Verification items for the finished model (mm, model axes). A direction names the side the tool comes from. Coordinates: 2 decimals unless noted, no trailing zeros. Write each loop counter-clockwise with the first axis right and the second up, starting at its lowest first coordinate (ties: lowest second). Pieces come first, ordered by that corner, then holes. Notation, with made-up numbers: M 47.5,61.5 L 79.5,61.5 A13 cw 79.5,81.5 Z; hole C -24.75,53 d11. An arc over 180 degrees is marked long. One line per item, written item: value.
Autodesk Inventor part; units mm, degrees
ref_plane "YZ Plane" through (0, 0, 0) normal (1, 0, 0) x (0, 1, 0)
ref_plane "XZ Plane" through (0, 0, 0) normal (0, 1, 0) x (-1, 0, 0)
ref_plane "XY Plane" through (0, 0, 0) normal (0, 0, 1) x (1, 0, 0)
sketch "Sketch1" plane through (0, 0, 0) normal (0, 0, 1) x (1, 0, 0)
  circle A0 centre (0, 0) radius 18.2563
  dimension "d0" = 36.5125
extrude "Extrusion1" add sketch "Sketch1" along normal blind 22.225
sketch "Sketch2" plane through (0, 0, 22.225) normal (0, 0, 1) x (1, 0, 0)
  circle A0 centre (0, 0) radius 18.2562
  circle A1 centre (0, 0) radius 17.4625
  dimension "d3" = 34.925
extrude "Extrusion2" add sketch "Sketch2" along normal blind 41.275 contours A1
fillet "Fillet1" radius 1.5875 1 edges at (-18.2563, 0, 0)
sketch "Sketch3" plane through (0, 0, 0) normal (0, 0, -1) x (-1, 0, 0)
  circle A0 centre (0, 0) radius 16.6687
  circle A1 centre (0, 7.9375) radius 6.35
  dimension "d7" = 12.7
  dimension "d8" = 7.9375
extrude "Extrusion3" add sketch "Sketch3" along normal blind 6.35 contours A1
sketch "Sketch4" plane through (0, 7.9375, -6.35) normal (0, 0, -1) x (-1, 0, 0)
  circle A0 centre (0, 0) radius 6.35
  circle A1 centre (0, 0) radius 3.175
  point P0 (0, -7.9375)
  dimension "d11" = 6.35
hole "Hole1" at (0, 7.9375, -6.35) direction (0, 0, 1) diameter 6.35 depth 6.35
properties part number "Motorbase"
Item 1: Cross-section at C-C, the plane z = 21.5. Enter the section's corners in (x, y).
The answers:
outline: C 0,0 d36.51
Item 2: Go/stop test with flat-tipped pins: P1, Ø6, axis at x = -11.5, z = 23.5, coming from the +Y side; P2, Ø3, axis at y = -3, z = 10, coming from the +X side; P3, Ø10, axis at x = 8.5, z = 44, coming from the -Y side. Record where each tip stops, or that it passes through.
The answers:
P1: stops at y = 16
P2: stops at x = 18.19
P3: stops at y = -17.11
Item 3: Cross-section at B-B, the plane y = 0. Enter the section's corners in (x, z) (1 decimal), and give its area (3 significant figures).
The answers:
outline: M -18.3,1.6 A1.6 ccw -16.7,0 L 16.7,0 A1.6 ccw 18.3,1.6 L 18.3,22.2 L 17.5,22.2 L 17.5,63.5 L -17.5,63.5 L -17.5,22.2 L -18.3,22.2 Z
area: 2,250 mm²
Item 4: Access from +Z, -Z, +X, -X, +Y, -Y to the whole of each face (thin tool, end or side, straight path). Record for faces 1 (the face through (-0.954, 10.966, -3.131)), 2 (the face through (2, 11, -6.35)).
The answers:
face 1: -Z
face 2: -Z, +X, -X, +Y, -Y
Item 5: Draft check along X on faces 3 (the face through (0, 0, 63.5)), 4 (the face through (-13.858, 10.626, 42.574)), 5 (the face through (0, 8, 0)). Enter one of: released by +X, released by -X, zero draft, split by the parting line, or undercut.
The answers:
face 3: zero draft
face 4: split by the parting line
face 5: undercut
Item 6: Scan lines: line 1 (Y direction, x = 0, z = -3.5); line 2 (Z direction, x = -5.5, y = -3.5); line 3 (Y direction, x = 4.5, z = 18.5). Record each from-to range of solid material in increasing order.
The answers:
line 1: y = 1.59 to 4.76, 11.11 to 14.29
line 2: z = 0 to 63.5
line 3: y = -17.69 to 17.69
Item 7: Cross-section at D-D, the plane z = 36. Enter the section's corners in (x, y) (1 decimal).
The answers:
outline: C 0,0 d34.9
